Source: three-view drawing plus pictorial views. Frame: mm from the lowest corner of the part. Give positions to 0.01 mm unless a question says otherwise; leave off trailing zeros. Order: outer loops, then holes, each group sorted by start corner. A loop starts at its lowest first (then second) coordinate and runs counter-clockwise, first axis right, second up.
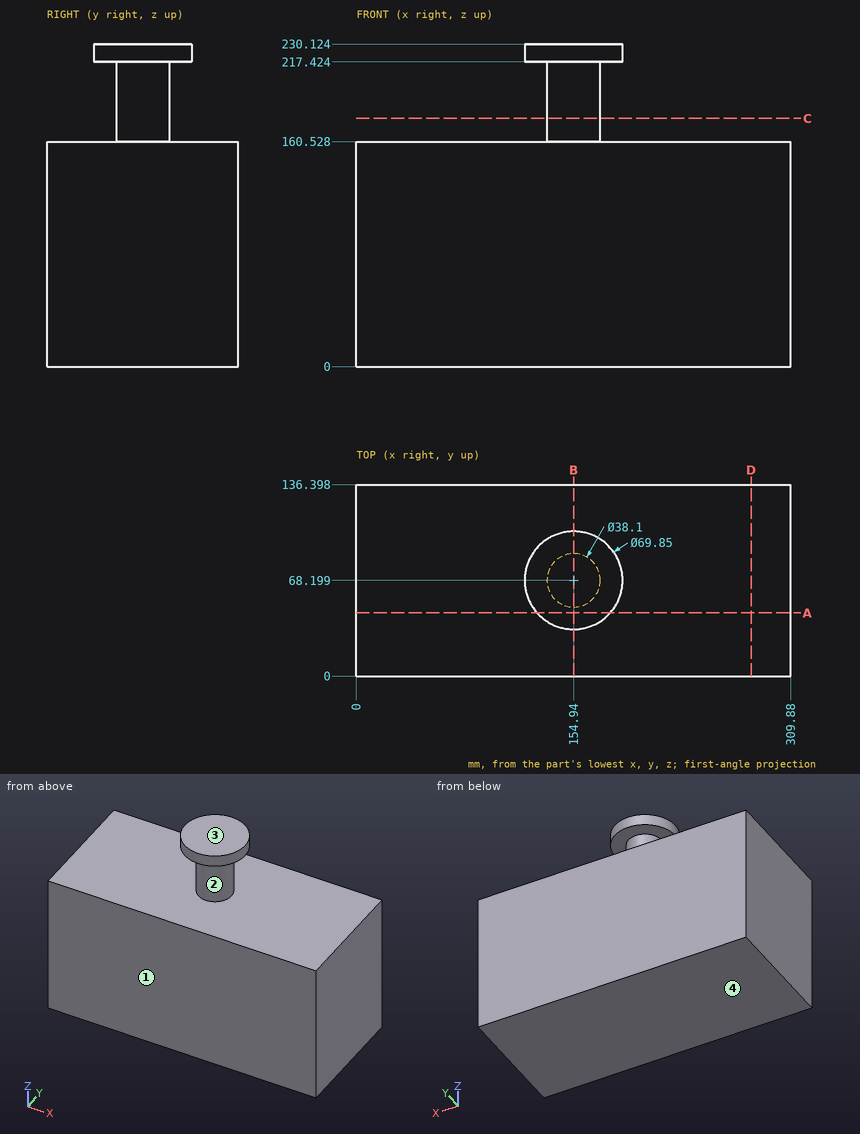
1) Section query B-B on x = 154.94. Output: boundary loops of the cut face in (y, z).
Checks:
outline: (0, 0) - (136.4, 0) - (136.4, 160.53) - (87.25, 160.53) - (87.25, 217.42) - (103.12, 217.42) - (103.12, 230.12) - (33.27, 230.12) - (33.27, 217.42) - (49.15, 217.42) - (49.15, 160.53) - (0, 160.53) - close
2) Section query A-A on y = 45. Output: boundary loops of the cut face in (x, z), and give its area (3 significant figures).
Checks:
outline: (0, 0) - (309.88, 0) - (309.88, 160.53) - (0, 160.53) - close; (128.83, 217.42) - (181.05, 217.42) - (181.05, 230.12) - (128.83, 230.12) - close
area: 50,400 mm2
3) Ray query, L1, parallel to Z at x = 232, y = 70; L2, parallel to Y at x = 146, z = 184.5. Return the intervals inside material, ascending.
Checks:
L1: z = 0 to 160.53
L2: y = 51.38 to 85.02
4) Pull-direction query (Z, two-part tool) for the marked faces 1, 2, 3 and 4; classes: +Z half, -Z half, draft (parallel to the pull), parting line (faces both ways), or undercut.
Checks:
face 1: draft
face 2: undercut
face 3: +Z half
face 4: -Z half
5) Section query D-D on x = 281.5. Output: boundary loops of the cut face in (y, z), and give its area (3 significant figures).
Checks:
outline: (0, 0) - (136.4, 0) - (136.4, 160.53) - (0, 160.53) - close
area: 21,900 mm2
6) Section query C-C on z = 177. Output: boundary loops of the cut face in (x, y), and give its area (3 significant figures).
Checks:
outline: circle Ø38.1 at (154.94, 68.2)
area: 1,140 mm2
7) First-contact query: pin 1 Ø1 at (x, y) = (169, 29.5) entering from +Z. Flat tip, straight axial feed; report the tip coordinate or a pass-through.
Checks:
pin 1: stops at z = 160.53
